Design review of the part built by this model. Coordinates are the model's own, in mm. Face numbers are marked on the shaded views. A direction names the side the tool comes from. Give positions to 0.01 mm unless a question says otherwise; leave off trailing zeros. Order: outer loops, then holes, each group sorted by start corner. A loop starts at its lowest first (then second) coordinate and runs counter-clockwise, first axis right, second up. Notation, with made-up numbers: (-29.75, 52.5) -> (-5.75, 52.5) arc R7 ccw to (-5.75, 60.5) -> close; hole circle Ø10 at (-4, 23.5). An arc over 180 degrees is marked (long way). One line per item, written item: value. Start each with the question number.
1) Wall thickness on line 1 along Y through (x, z) = (0, 92) (3 decimals); line 2 along Y through (x, z) = (0, 257) (3 decimals); line 3 along Z through (x, y) = (-3.5, 44): over which ranges is each line inside the solid? List them lowest first. Write a range as from..to.
2) Tool access review of the marked faces 1 and 2: name each direction out of +Z, -Z, +X, -X, +Y, -Y from which nothing blocks a thin tool from reaching the whole face with its end or side.
3) Consider section C-C (z = 416). State the section outline as (x, y) points (3 decimals).
4) For pin 1 (5 mm diameter, centred on x = -1.5, y = 21.5, fed in from -Z); pin 2 (6 mm diameter, centred on y = 12.5, z = 245.5, fed in from -X); pin 3 (10.5 mm diameter, centred on x = 0, y = 35, fed in from +Z); pin 4 (13 mm diameter, centred on x = -6.5, y = 13, fed in from -Z), all flat-tipped, find the tip position at first contact; note any pin that passes through.
5) Consider section B-B (x = 0). State the section outline as (y, z) points (3 decimals), plus the area to 3 significant figures.
6) Consider section A-A (y = 0). State the section outline as (x, z) points (3 decimals).
7) Consider section D-D (y = 18). State the section outline as (x, z) points.
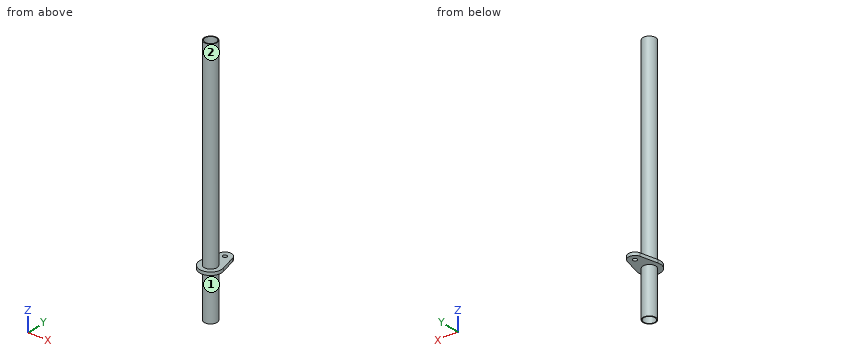
from build123d import *

# Parameters (mm, degrees)
SKETCH1_R           = 12.525
SKETCH1_R_2         = 11.025
EXTRUDE_THIN1_DEPTH = 490
BOSS_EXTRUDE2_START = 90
SKETCH1_4_R         = 12.525
SKETCH1_4_R_2       = 4.025
BOSS_EXTRUDE2_DEPTH = 6


with BuildPart() as part:
    # Sketch1 → Extrude-Thin1 (new body)
    with BuildSketch(Plane.XY):
        Circle(SKETCH1_R)
        Circle(SKETCH1_R_2, mode=Mode.SUBTRACT)
    extrude(amount=EXTRUDE_THIN1_DEPTH)

    # Sketch1_4 → Boss-Extrude2 (add)
    with BuildSketch(Plane.XY.offset(BOSS_EXTRUDE2_START)):
        with BuildLine():
            Line((-20.880585929, 5.2275), (-12.635058385, 38.163214286))
            ThreePointArc((-12.635058385, 38.163214286), (0, 48.025), (12.635058385, 38.163214286))
            Line((12.635058385, 38.163214286), (20.880585929, 5.2275))
            ThreePointArc((20.880585929, 5.2275), (0, -21.525), (-20.880585929, 5.2275))
        make_face()
        with Locations(Location((0, 0, 0), (0, 0, 180))):
            Circle(SKETCH1_4_R, mode=Mode.SUBTRACT)
        with Locations((0, 35)):
            Circle(SKETCH1_4_R_2, mode=Mode.SUBTRACT)
    extrude(amount=BOSS_EXTRUDE2_DEPTH)


solid = part.part
Checked values:
1. line 1: y = -21.525..-11.025, 11.025..30.975, 39.025..48.025
1. line 2: y = -12.525..-11.025, 11.025..12.525
1. line 3: z = 90..96
2. face 1: -Z
2. face 2: +Z
3. outline: circle Ø25.05 at (0, 0); hole circle Ø22.05 at (0, 0)
4. pin 1: stops at z = 90
4. pin 2: stops at x = -8.16
4. pin 3: stops at z = 96
4. pin 4: stops at z = 0
5. outline: (-21.525, 90) -> (-12.525, 90) -> (-12.525, 0) -> (-11.025, 0) -> (-11.025, 490) -> (-12.525, 490) -> (-12.525, 96) -> (-21.525, 96) -> close; (11.025, 0) -> (12.525, 0) -> (12.525, 90) -> (30.975, 90) -> (30.975, 96) -> (12.525, 96) -> (12.525, 490) -> (11.025, 490) -> close; (39.025, 90) -> (48.025, 90) -> (48.025, 96) -> (39.025, 96) -> close
5. area: 1,690 mm^2
6. outline: (-21.525, 90) -> (-12.525, 90) -> (-12.525, 0) -> (-11.025, 0) -> (-11.025, 490) -> (-12.525, 490) -> (-12.525, 96) -> (-21.525, 96) -> close; (11.025, 0) -> (12.525, 0) -> (12.525, 90) -> (21.525, 90) -> (21.525, 96) -> (12.525, 96) -> (12.525, 490) -> (11.025, 490) -> close
7. outline: (-17.68, 90) -> (17.68, 90) -> (17.68, 96) -> (-17.68, 96) -> close
